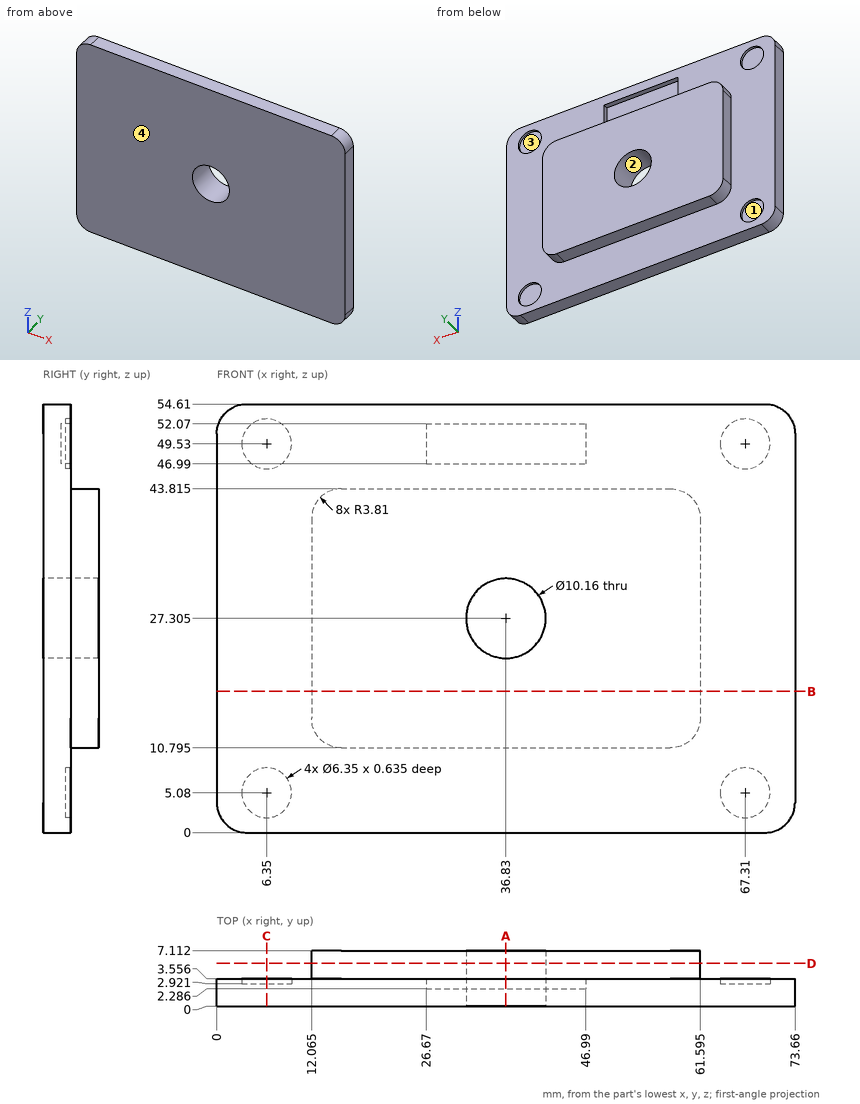
Input: dimensioned drawing with shaded views. Units: mm. Origin: part minimum x, y, z. A direction names the side the tool comes from. Round coordinates to 2 decimals unless told otherwise and drop trailing zeros. Loops run counter-clockwise (first coordinate to the right, second up) from the corner with the lowest first, then second, coordinate; pieces in that order, holes last.
1) Set-up query: the marked faces 1 and 2. Return all of +Z, -Z, +X, -X, +Y, -Y with unobstructed straight access to the full face (end or side cutting, diameter ignored); none if empty.
Ans:
face 1: +Y
face 2: +Y, -Y
2) Section query D-D on y = 5.5. Return the cut outline in (x, z) (3 decimals), plus the area to 3 significant figures.
Ans:
outline: (12.065, 14.605) arc R3.81 ccw to (15.875, 10.795) - (57.785, 10.795) arc R3.81 ccw to (61.595, 14.605) - (61.595, 40.005) arc R3.81 ccw to (57.785, 43.815) - (15.875, 43.815) arc R3.81 ccw to (12.065, 40.005) - close; hole circle Ø10.16 at (36.83, 27.305)
area: 1,540 mm2
3) Material intervals for line 1 (X direction, y = 3.4, z = 49.53) (3 decimals); line 2 (Z direction, x = 67.31, y = 3.1) (3 decimals); line 3 (X direction, y = 3.2, z = 5.08) (3 decimals), sorted ascending.
Ans:
line 1: x = 0 to 3.175, 9.525 to 26.67, 46.99 to 64.135, 70.485 to 73.66
line 2: z = 0 to 1.905, 8.255 to 46.355, 52.705 to 54.61
line 3: x = 0 to 3.175, 9.525 to 64.135, 70.485 to 73.66
4) Pin query (flat end, axial travel): pin 1 (8.5 mm diameter, centred on x = 6.35, z = 5.08, fed in from +Y); pin 2 (1.8 mm diameter, centred on x = 27.5, y = 5.5, fed in from -Z) (3 decimals); pin 3 (1.8 mm diameter, centred on x = 39.5, y = 4.5, fed in from +Z) (3 decimals); pin 4 (6 mm diameter, centred on x = 36.83, z = 27.305, fed in from +Y). Return the tip coordinate at first contact, or that it passes through.
Ans:
pin 1: stops at y = 3.56
pin 2: stops at z = 10.795
pin 3: stops at z = 43.815
pin 4: passes through
5) Section query C-C on x = 6.35. Return the cut outline in (y, z) (3 decimals).
Ans:
outline: (0, 0) - (3.556, 0) - (3.556, 1.905) - (2.921, 1.905) - (2.921, 8.255) - (3.556, 8.255) - (3.556, 46.355) - (2.921, 46.355) - (2.921, 52.705) - (3.556, 52.705) - (3.556, 54.61) - (0, 54.61) - close
6) Section query B-B on z = 18. Return the cut outline in (x, y) (3 decimals), plus the area to 3 significant figures.
Ans:
outline: (0, 0) - (73.66, 0) - (73.66, 3.556) - (61.595, 3.556) - (61.595, 7.112) - (12.065, 7.112) - (12.065, 3.556) - (0, 3.556) - close
area: 438 mm2
7) Pull-direction query (X, two-part tool) for the marked faces 3 and 4; classes: released by +X, released by -X, zero draft, split by the parting line, or undercut.
Ans:
face 3: undercut
face 4: zero draft
8) Section query A-A on x = 36.83. Return the cut outline in (y, z) (3 decimals), plus the area to 3 significant figures.
Ans:
outline: (0, 0) - (3.556, 0) - (3.556, 10.795) - (7.112, 10.795) - (7.112, 22.225) - (0, 22.225) - close; (0, 32.385) - (7.112, 32.385) - (7.112, 43.815) - (3.556, 43.815) - (3.556, 46.99) - (2.286, 46.99) - (2.286, 52.07) - (3.556, 52.07) - (3.556, 54.61) - (0, 54.61) - close
area: 233 mm2
